Verification items for the finished model (mm, model axes). Give positions to 0.01 mm unless a question says otherwise; leave off trailing zeros. Loops run counter-clockwise (first coordinate to the right, second up) from the corner with the lowest first, then second, coordinate; pieces in that order, holes last. Notation, with made-up numbers: M 79.5,87.5 L 113.5,87.5 A16 cw 113.5,100.5 Z; hole C 22.25,80.25 d4. An arc over 180 degrees is marked long. Use a Markdown table: item, result.
Autodesk Inventor part; units mm, degrees
ref_plane "YZ Plane" through (0, 0, 0) normal (1, 0, 0) x (0, 1, 0)
ref_plane "XZ Plane" through (0, 0, 0) normal (0, 1, 0) x (-1, 0, 0)
ref_plane "XY Plane" through (0, 0, 0) normal (0, 0, 1) x (1, 0, 0)
sketch "Sketch1" plane through (0, 0, 0) normal (0, 0, 1) x (1, 0, 0)
  circle A0 centre (0, 0) radius 107.5
  dimension "d0" = 215
extrude "Extrusion1" add sketch "Sketch1" along normal blind 1.6
sketch "Sketch2" plane through (0, 0, 1.6) normal (0, 0, 1) x (1, 0, 0)
  circle A0 centre (0, 0) radius 107.5
  line L0 (0, 102.5) -> (0, 0) construction
  dimension "d3" = 102.5
hole "Hole1" at (0, 102.5, 1.6) direction (0, 0, -1) diameter 3 end through all
pattern_circular "Circular Pattern1" count 3 over 360 about axis through (0, 0, 0) along (0, 0, 1) of "Hole1"
sketch "Sketch3" plane through (0, 0, 1.6) normal (0, 0, 1) x (1, 0, 0)
  circle A0 centre (0, 0) radius 107.5
  line L0 (-17.5, -93.495) -> (-17.5, -100.995) construction
  line L1 (-20, -93.495) -> (-20, -100.995)
  line L2 (-15, -100.995) -> (-15, -93.495)
  arc A1 (-15, -93.495) -> (-20, -93.495) centre (-17.5, -93.495) ccw
  arc A2 (-20, -100.995) -> (-15, -100.995) centre (-17.5, -100.995) ccw
  line L3 (5, -94.9305) -> (5, -102.4305) construction
  line L4 (2.5, -94.9305) -> (2.5, -102.4305)
  line L5 (7.5, -102.4305) -> (7.5, -94.9305)
  arc A3 (7.5, -94.9305) -> (2.5, -94.9305) centre (5, -94.9305) ccw
  arc A4 (2.5, -102.4305) -> (7.5, -102.4305) centre (5, -102.4305) ccw
  line L6 (17.5, -93.495) -> (17.5, -100.995) construction
  line L7 (15, -93.495) -> (15, -100.995)
  line L8 (20, -100.995) -> (20, -93.495)
  arc A5 (20, -93.495) -> (15, -93.495) centre (17.5, -93.495) ccw
  arc A6 (15, -100.995) -> (20, -100.995) centre (17.5, -100.995) ccw
  arc A7 (-17.5, -97.245) -> (17.5, -97.245) centre (0, 0) ccw construction
  line L9 (-17.5, -97.245) -> (17.5, -97.245) construction
  point P0 (5, -98.6805)
  dimension "d14" = 7.5
  dimension "d15" = 2.5
  dimension "d16" = 35
  dimension "d17" = 2.5
  dimension "d18" = 12.5
extrude "Extrusion2" add sketch "Sketch3" along normal blind 0.5 draft -10 contours A1 L2 A2 L1 | A3 L5 A4 L4 | A5 L8 A6 L7
properties part number "Heatbed_Geeetech_215mm"
(1) Cross-section at B-B on z = 0.75. Record the cut outline in (x, y), then the cut area to 3 significant figures.
Results below:
| item | result |
|---|---|
| outline | C 0,0 d215; hole C -88.77,-51.25 d3; hole C 0,102.5 d3; hole C 88.77,-51.25 d3 |
| area | 36,300 mm^2 |
(2) Cross-section at C-C on x = -28. Record the cut outline in (y, z).
Results below:
| item | result |
|---|---|
| outline | M -103.79,0 L 103.79,0 L 103.79,1.6 L -103.79,1.6 Z |
(3) Gauge pin test, flat end, axial feed: P1, Ø1, axis at x = 11, y = 54, coming from the +Z side. Record the tip position at first contact, or that the pin passes through.
Results below:
| item | result |
|---|---|
| P1 | z = 1.6 |
(4) Cross-section at A-A on y = 0. Record the cut outline in (x, z).
Results below:
| item | result |
|---|---|
| outline | M -107.5,0 L 107.5,0 L 107.5,1.6 L -107.5,1.6 Z |
(5) Material ranges on line 1 (X direction, y = -99, z = 1.8); line 2 (Y direction, x = 0, z = 0.85); line 3 (X direction, y = -51.25, z = 0.95), recorded low to high.
Results below:
| item | result |
|---|---|
| line 1 | -19.96 to -15.04, 2.54 to 7.46, 15.04 to 19.96 |
| line 2 | -107.5 to 101, 104 to 107.5 |
| line 3 | -94.5 to -90.27, -87.27 to 87.27, 90.27 to 94.5 |
